Input: part model. Units: mm. Frame: model coordinates. A direction names the side the tool comes from. Give positions to 0.01 mm unless a question says otherwise; leave off trailing zeros. Write each loop counter-clockwise with the first axis right and the second up, starting at its lowest first coordinate (ties: lowest second). Pieces come first, ordered by that corner, then holes. Notation, with made-up numbers: (70.25, 16) - (97.25, 16) arc R18 ccw to (97.25, 38) - close; hole circle Ø4 at (65.25, -24). An arc over 180 degrees is marked (long way). Answer as CSV lines item,"result".
```python
from build123d import *

# Parameters (mm, degrees)
F0_R     = 25.4
F1_DEPTH = 12.7


# Not quite as in the source:
# - a length typed as a fraction of an inch, garbled in the dataset ("3 / 203.2 mm" for 3/8 in), is restored


with BuildPart() as f1:
    # F0 (on Front) → F1 (new body)
    with BuildSketch(Plane.XZ):
        Polygon((-3.9472851508, 53.245825498), (-96.0222851508, 53.245825498), (-96.0222851508, -73.754174502), (81.7777148492, -73.754174502), (81.7777148492, 53.245825498), (65.9027148492, 53.245825498), (65.9027148492, -22.954174502), (-3.9472851508, -22.954174502), align=None)
        with Locations((-45.2222851508, -22.954174502)):
            Circle(F0_R, mode=Mode.SUBTRACT)
    extrude(amount=F1_DEPTH)


solid = f1.part
```
Item 1: Reachability of faces 1 (the face through (-3.947, -6, 15)), 2 (the face through (-8, -12.7, -9)) from +Z, -Z, +X, -X, +Y, -Y: full face, straight path, thin tool, end or side. Return the list, or none.
The answers:
face 1,"+Z, +Y, -Y"
face 2,"+Z, -Z, +X, -X, -Y"
Item 2: Cut plane A-A on y = -4.5. Return the cut outline in (x, z), plus the area to 3 significant figures.
The answers:
outline,"(-96.02, -73.75) - (81.78, -73.75) - (81.78, 53.25) - (65.9, 53.25) - (65.9, -22.95) - (-3.95, -22.95) - (-3.95, 53.25) - (-96.02, 53.25) - close; hole circle Ø50.8 at (-45.22, -22.95)"
area,"15,200 mm²"
Item 3: Cut plane C-C on z = -15. Return the cut outline in (x, y).
The answers:
outline,"(-96.02, -12.7) - (-69.34, -12.7) - (-69.34, 0) - (-96.02, 0) - close; (-21.1, -12.7) - (-3.95, -12.7) - (-3.95, 0) - (-21.1, 0) - close; (65.9, -12.7) - (81.78, -12.7) - (81.78, 0) - (65.9, 0) - close"
Item 4: Cut plane D-D on x = 16. Return the cut outline in (y, z).
The answers:
outline,"(-12.7, -73.75) - (0, -73.75) - (0, -22.95) - (-12.7, -22.95) - close"
Item 5: Mould query, pull axis X, two halves, no side actions, for faces 3 (the face through (-8, -6, -73.754)), 4 (the face through (81.778, -6, -11)), 5 (the face through (-21.76, -6.26, -32.68)), 6 (the face through (-96.022, -6, -9)). Classes: +X half, -X half, draft (parallel to the pull), parting line (faces both ways), or undercut.
The answers:
face 3,"draft"
face 4,"+X half"
face 5,"undercut"
face 6,"-X half"
Item 6: Ray query, line 1 (X direction, y = -6.75, z = -22.5); line 2 (X direction, y = -9, z = -20.5); line 3 (X direction, y = -8.5, z = 8). Return the intervals inside material, ascending. Write a range as from..to.
The answers:
line 1,"-96.02..-70.62, -19.83..-3.95, 65.9..81.78"
line 2,"-96.02..-70.5, -19.94..-3.95, 65.9..81.78"
line 3,"-96.02..-3.95, 65.9..81.78"
Item 7: Contact query for a flat-ended pin moving along its axis: pin 1 (5 mm diameter, centred on x = 61.5, y = -6, fed in from +Z). Output: stop coordinate, or through.
The answers:
pin 1,"z = -22.95"
Item 8: Cut plane B-B on z = 5. Return the cut outline in (x, y).
The answers:
outline,"(-96.02, -12.7) - (-3.95, -12.7) - (-3.95, 0) - (-96.02, 0) - close; (65.9, -12.7) - (81.78, -12.7) - (81.78, 0) - (65.9, 0) - close"
